```python
from build123d import *

# Parameters (mm, degrees)
F0_R     = 34.925
F1_DEPTH = 152.4
F2_R     = 19.05
F3_DEPTH = 44.45
F4_R     = 19.05
F5_DEPTH = 44.45
F6_R     = 3.175
F7_DEPTH = 152.4


with BuildPart() as f1:
    # F0 (on Top) → F1 (new body)
    with BuildSketch(Plane.XY):
        Circle(F0_R)
    extrude(amount=F1_DEPTH)

    # F2 (on face) → F3 (cut)
    with BuildSketch(Plane.XY.offset(152.4)):
        Circle(F2_R)
    extrude(amount=-F3_DEPTH, mode=Mode.SUBTRACT)

    # F4 (on face) → F5 (cut)
    with BuildSketch(Plane(origin=(0, 0, 0), x_dir=(1, 0, 0), z_dir=(0, 0, -1))):
        Circle(F4_R)
    extrude(amount=-F5_DEPTH, mode=Mode.SUBTRACT)

    # F6 (on face) → F7 (cut)
    with BuildSketch(Plane.XY.offset(107.95)):
        Circle(F6_R)
    extrude(amount=-F7_DEPTH, mode=Mode.SUBTRACT)


solid = f1.part
```
Could you check a few things on this model? Use its own coordinates, in mm. A direction names the side the tool comes from. Give positions to 0.01 mm unless a question says otherwise; leave off trailing zeros. Loops run counter-clockwise (first coordinate to the right, second up) from the corner with the lowest first, then second, coordinate; pieces in that order, holes last. Notation, with made-up numbers: (81.25, 74) - (104.25, 74) arc R9 cw to (104.25, 91) - close; hole circle Ø1 at (78.5, 42.25). An arc over 180 degrees is marked (long way). Answer in a Markdown table with one row per item. Add a question column.
Q1. If we section it at D-D (y = 9.5): List the corners of the cut face in (x, z) for me, plus the area to 3 significant figures.
Q2. We'd pull the mould along X, two halves only. Please class faces 4 (the face through (-27.715, -21.251, 75.133)), 5 (the face through (-15.12, 11.59, 21.91)), 6 (the face through (15, -15, 152.4)): +X half, -X half, draft (parallel to the pull), parting line (faces both ways), or undercut.
Q3. For pin 1 (5 mm diameter, centred on x = 13, z = 21.5, fed in from -Y); pin 2 (10 mm diameter, centred on x = 0, y = 0, fed in from +Z); pin 3 (12 mm diameter, centred on y = 4.5, z = 93.5, fed in from +X) (3 decimals); pin 4 (1.5 mm diameter, centred on y = 25.5, z = 49.5, fed in from -X), each with a flat end and sliding along its axis, tell me the tip position at first contact or that it passes through.
Q4. Please list where these lines run through material, in increasing order: L1, parallel to Y at x = 0, z = 90.5 (3 decimals); L2, parallel to Z at x = -13, y = 12; L3, parallel to Y at x = 0, z = 139 (3 decimals). Write a range as from..to.
Q5. If we section it at A-A (y = 0): List the corners of the cut face in (x, z) for me (3 decimals).
Q6. Which directions (+Z, -Z, +X, -X, +Y, -Y) give clear straight access to the entire face, cutting with the end or side of a thin tool? Please do faces 1 (the face through (4, 0, 44.45)), 2 (the face through (-15.12, -11.59, 130.49)), 3 (the face through (-0.69, -3.1, 76.64)).
Q7. If we section it at C-C (z = 113.5): List the corners of the cut face in (x, y) for me (3 decimals), plus the area to 3 significant figures.
The answers:
| question | item | result |
|---|---|---|
| 1 | outline | (-33.61, 0) - (-16.51, 0) - (-16.51, 44.45) - (16.51, 44.45) - (16.51, 0) - (33.61, 0) - (33.61, 152.4) - (16.51, 152.4) - (16.51, 107.95) - (-16.51, 107.95) - (-16.51, 152.4) - (-33.61, 152.4) - close |
| 1 | area | 7,310 mm^2 |
| 2 | face 4 | parting line |
| 2 | face 5 | undercut |
| 2 | face 6 | draft |
| 3 | pin 1 | stops at y = -33.31 |
| 3 | pin 2 | stops at z = 107.95 |
| 3 | pin 3 | stops at x = 34.925 |
| 3 | pin 4 | stops at x = -24.64 |
| 4 | L1 | y = -34.925..-3.175, 3.175..34.925 |
| 4 | L2 | z = 44.45..107.95 |
| 4 | L3 | y = -34.925..-19.05, 19.05..34.925 |
| 5 | outline | (-34.925, 0) - (-19.05, 0) - (-19.05, 44.45) - (-3.175, 44.45) - (-3.175, 107.95) - (-19.05, 107.95) - (-19.05, 152.4) - (-34.925, 152.4) - close; (3.175, 44.45) - (19.05, 44.45) - (19.05, 0) - (34.925, 0) - (34.925, 152.4) - (19.05, 152.4) - (19.05, 107.95) - (3.175, 107.95) - close |
| 6 | face 1 | -Z |
| 6 | face 2 | +Z |
| 6 | face 3 | +Z, -Z |
| 7 | outline | circle Ø69.85 at (0, 0); hole circle Ø38.1 at (0, 0) |
| 7 | area | 2,690 mm^2 |
